from build123d import *

# Parameters (mm, degrees)
F0_R      = 19.75
F1_DEPTH  = 17
F2_R      = 18.25
F3_DEPTH  = 15
F4_R      = 9.5
F5_DEPTH  = 14.5
F6_R      = 7.662352
F7_DEPTH  = 14
F8_R      = 3.1
F9_DEPTH  = 9.5
F10_R     = 1.640343
F11_DEPTH = 7
F12_R     = 1.631473
F13_DEPTH = 25.4
F14_R     = 3
F15_DEPTH = 2
F16_R     = 1.75
F17_DEPTH = 2
F18_R     = 0.4
F19_DEPTH = 1
F20_R     = 1


with BuildPart() as f1:
    # F0 (on Front) → F1 (new body)
    with BuildSketch(Plane.XZ):
        Circle(F0_R)
    extrude(amount=F1_DEPTH)

    # F2 (on face) → F3 (cut)
    with BuildSketch(Plane.XZ.offset(17)):
        Circle(F2_R)
    extrude(amount=-F3_DEPTH, mode=Mode.SUBTRACT)

    # F4 (on face) → F5 (join)
    with BuildSketch(Plane(origin=(0, 0, 0), x_dir=(-1, 0, 0), z_dir=(0, 1, 0))):
        Circle(F4_R)
    extrude(amount=-F5_DEPTH)

    # F6 (on face) → F7 (cut)
    with BuildSketch(Plane(origin=(0, 0, 0), x_dir=(-1, 0, 0), z_dir=(0, 1, 0))):
        Circle(F6_R)
    extrude(amount=-F7_DEPTH, mode=Mode.SUBTRACT)

    # F8 (on face) → F9 (join)
    with BuildSketch(Plane.XZ.offset(14.5)):
        Circle(F8_R)
    extrude(amount=F9_DEPTH)

    # F10 (on face) → F11 (cut)
    with BuildSketch(Plane.XZ.offset(24)):
        Circle(F10_R)
    extrude(amount=-F11_DEPTH, mode=Mode.SUBTRACT)

    # F12 (on face) → F13 (cut)
    with BuildSketch(Plane(origin=(0, -14, 0), x_dir=(-1, 0, 0), z_dir=(0, 1, 0))):
        with Locations((-2.547523, 4.201843)):
            Circle(F12_R)
        with Locations((1.169781, 4.772522)):
            Circle(F12_R)
        with Locations((4.201843, 2.547523)):
            Circle(F12_R)
        with Locations((4.772522, -1.169781)):
            Circle(F12_R)
        with Locations((2.547523, -4.201843)):
            Circle(F12_R)
        with Locations((-1.169781, -4.772522)):
            Circle(F12_R)
        with Locations((-4.201843, -2.547523)):
            Circle(F12_R)
        with Locations((-4.772522, 1.169781)):
            Circle(F12_R)
    extrude(amount=-F13_DEPTH, mode=Mode.SUBTRACT)

    # F14 (on face) → F15 (join)
    with BuildSketch(Plane(origin=(0, -14, 0), x_dir=(-1, 0, 0), z_dir=(0, 1, 0))):
        Circle(F14_R)
    extrude(amount=F15_DEPTH)

    # F16 (on face) → F17 (join)
    with BuildSketch(Plane(origin=(0, -12, 0), x_dir=(-1, 0, 0), z_dir=(0, 1, 0))):
        Circle(F16_R)
    extrude(amount=F17_DEPTH)

    # F18 (on face) → F19 (join)
    with BuildSketch(Plane(origin=(0, -12, 0), x_dir=(-1, 0, 0), z_dir=(0, 1, 0))):
        with Locations((0.285372, 2.338507)):
            Circle(F18_R)
        with Locations((1.60541, 1.724155)):
            Circle(F18_R)
        with Locations((2.312237, 0.451234)):
            Circle(F18_R)
        with Locations((2.135868, -0.994043)):
            Circle(F18_R)
        with Locations((1.14367, -2.059629)):
            Circle(F18_R)
        with Locations((-0.285372, -2.338507)):
            Circle(F18_R)
        with Locations((-2.312237, -0.451234)):
            Circle(F18_R)
        with Locations((-1.14367, 2.059629)):
            Circle(F18_R)
        with Locations((-2.135868, 0.994043)):
            Circle(F18_R)
        with Locations((-1.60541, -1.724155)):
            Circle(F18_R)
    extrude(amount=F19_DEPTH)

    # F20
    f20_edges = [f1.edges().sort_by_distance(p)[0] for p in [
        (-19.75, 0, 0),
    ]]
    fillet(f20_edges, radius=F20_R)


solid = f1.part
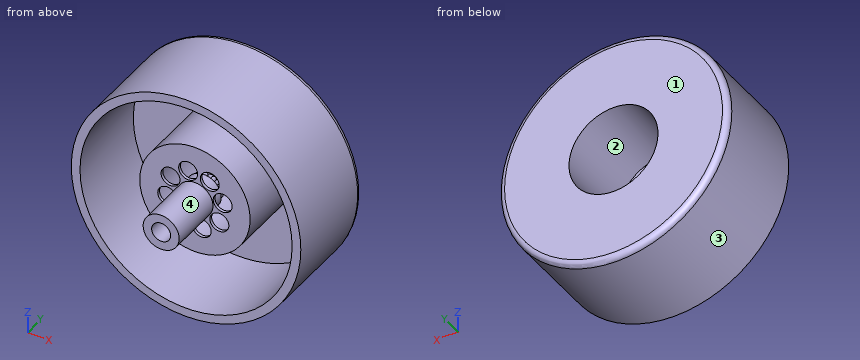
Check sheet for the modelled part. Datum: model origin and axes. Units: mm. Face numbers are marked on the shaded views. Round coordinates to 2 decimals unless told otherwise and drop trailing zeros. Loops run counter-clockwise (first coordinate to the right, second up) from the corner with the lowest first, then second, coordinate; pieces in that order, holes last.
1. Sectioned sample at A-A on y = -6.25. Record the boundary of the cut face in (x, z), and give its area (3 significant figures).
2. Sectioned sample at B-B on y = -19.5. Record the boundary of the cut face in (x, z).
3. Mould release check, pull along X, two halves, no side actions. Record for the marked faces 1, 2, 3 and 4: released by +X, released by -X, zero draft, split by the parting line, or undercut.
4. Gauge pin test, flat ends, axial feed: pin 1 Ø0.9 at (x, z) = (-2.5, 0.5) entering from +Y; pin 2 Ø8 at (x, y) = (2.5, -3) entering from +Z; pin 3 Ø5 at (y, z) = (-6, -15) entering from -X; pin 4 Ø4 at (y, z) = (-19.5, 14) entering from -X. Record the tip position at first contact, or that the pin passes through.
5. Scan lines: probe 1 along Z at (x, y) = (0, -22); probe 2 along Z at (x, y) = (4.5, -10); probe 3 along Z at (x, y) = (-1.5, -16). Record each from-to range of solid material in increasing order.
Recorded:
1. outline: circle Ø39.5 at (0, 0); circle Ø19 at (0, 0); hole circle Ø36.5 at (0, 0); hole circle Ø15.32 at (0, 0)
1. area: 278 mm2
2. outline: circle Ø6.2 at (0, 0); hole circle Ø3.28 at (0, 0)
3. face 1: zero draft
3. face 2: undercut
3. face 3: split by the parting line
3. face 4: undercut
4. pin 1: stops at y = -11
4. pin 2: stops at z = 19.75
4. pin 3: stops at x = -15.29
4. pin 4: passes through
5. probe 1: z = -3.1 to -1.64, 1.64 to 3.1
5. probe 2: z = -19.23 to -17.69, -8.37 to -6.2, 6.2 to 8.37, 17.69 to 19.23
5. probe 3: z = -19.69 to -18.19, -2.71 to 2.71, 18.19 to 19.69
